```python
from build123d import *

# Parameters (mm, degrees)
ESQUISSE1_W                = 45
ESQUISSE1_H                = 13
BOSS_EXTRU_1_DEPTH         = 3
ESQUISSE2_R                = 1.5
ENL_V_MAT_EXTRU_1_DEPTH    = 4
BOSS_EXTRU_3_DEPTH         = 100
CONG_1_R                   = 1
ESQUISSE12_R               = 2.25
ENL_V_MAT_EXTRU_3_DEPTH    = 11.149508308
R_P_TITION_LIN_AIRE1_COUNT = 2
R_P_TITION_LIN_AIRE1_PITCH = 16


with BuildPart() as part:
    # Esquisse1 → Boss.-Extru.1 (new body)
    with BuildSketch(Plane.XY):
        with Locations((22.5, 6.5)):
            Rectangle(ESQUISSE1_W, ESQUISSE1_H)
    extrude(amount=BOSS_EXTRU_1_DEPTH)

    # Esquisse2 → Enl_v. mat.-Extru.1 (cut, through all)
    with BuildSketch(Plane.XY.offset(3)):
        with Locations((41, 6.5)):
            Circle(ESQUISSE2_R)
    enl_v_mat_extru_1 = extrude(amount=-ENL_V_MAT_EXTRU_1_DEPTH, mode=Mode.SUBTRACT)

    # Sym_trie1: Enl_v. mat.-Extru.1 across plane
    add(enl_v_mat_extru_1.mirror(Plane.ZY.offset(-22.5)), mode=Mode.SUBTRACT)

    # Esquisse8 → Boss.-Extru.3 (add)
    with BuildSketch(Plane.ZY):
        Polygon((0, 13), (-3.069268098, 21.432744793), (-0.420201433, 22.396926208), (3, 13), align=None)
    extrude(amount=-BOSS_EXTRU_3_DEPTH)

    # Cong_1
    cong_1_edges = [part.edges().sort_by_distance(p)[0] for p in [
        (45, 0, 1.5),
        (0, 0, 1.5),
        (45, 13, 1.5),
        (100, 13, 1.5),
        (100, 21.914835501, -1.744734766),
        (0, 21.914835501, -1.744734766),
    ]]
    fillet(cong_1_edges, radius=CONG_1_R)

    # Esquisse12 → Enl_v. mat.-Extru.3 (cut, through all)
    with BuildSketch(Plane(origin=(0, 2.484892534, 6.827186128), x_dir=(1, 0, 0), z_dir=(0, 0.342020143, 0.939692621))):
        with Locations((95, 15.68994364)):
            Circle(ESQUISSE12_R)
    enl_v_mat_extru_3 = extrude(amount=-ENL_V_MAT_EXTRU_3_DEPTH, mode=Mode.SUBTRACT)

    # R_p_tition lin_aire1: Enl_v. mat.-Extru.3 ×2
    with Locations(*[(-i * R_P_TITION_LIN_AIRE1_PITCH, 0, 0) for i in range(1, R_P_TITION_LIN_AIRE1_COUNT)]):
        add(enl_v_mat_extru_3, mode=Mode.SUBTRACT)


solid = part.part
```
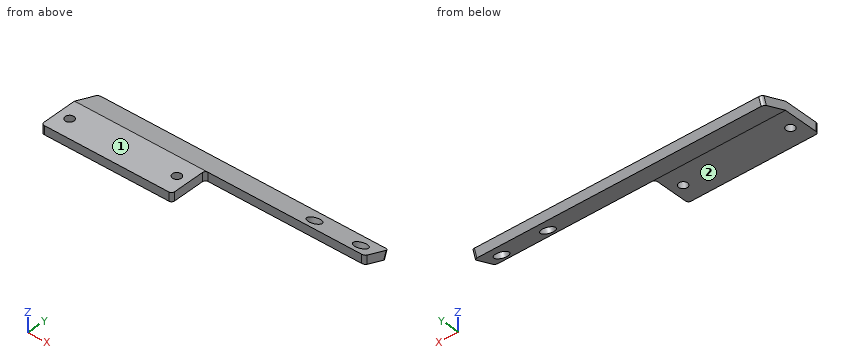
Part model, mm, in its own coordinate system. Face numbers are marked on the shaded views. A direction names the side the tool comes from. Coordinates: 2 decimals unless noted, no trailing zeros. Order: outer loops, then holes, each group sorted by start corner. A loop starts at its lowest first (then second) coordinate and runs counter-clockwise, first axis right, second up. Notation, with made-up numbers: (-20, 38.5) -> (7, 38.5) arc R38 cw to (7, 77.5) -> close; hole circle Ø5 at (-39, 30). An arc over 180 degrees is marked (long way). Put each result on its own line as item: value. Start each with the question number.
(1) Probe line 1 along X through (y, z) = (16.5, 1.25); line 2 along X through (y, z) = (11, 1.75); line 3 along Z through (x, y) = (9, 3). List the from-to ranges inside material, lowest first. Write a range as [from, to].
(2) Pin check, flat tips, straight feed: pin 1 Ø3.5 at (y, z) = (6.5, 1) entering from +X; pin 2 Ø1.5 at (x, y) = (26.5, 8) entering from -Z; pin 3 Ø2.5 at (x, z) = (69, 1.5) entering from -Y; pin 4 Ø1.8 at (x, y) = (41, 6.5) entering from +Z. Stop position of each tip, or through.
(3) Band-saw the part on B-B (y = 6.5). Give the cut face in (x, z), then the cut area to 3 significant figures.
(4) Band-saw the part on C-C (x = 86). Give the cut face in (y, z).
(5) Band-saw the part on A-A (x = 4). Give the cut face in (y, z).
(6) Which spindle directions (+Z, -Z, +X, -X, +Y, -Y) get a long thin tool onto all of the face, cutting with end or side? Do the marked faces 1 and 2. Say none if no direction does.
Determined:
1. line 1: x = [0, 76.83], [81.17, 92.83], [97.17, 100]
1. line 2: x = [0, 45]
1. line 3: z = [0, 3]
2. pin 1: stops at x = 45
2. pin 2: stops at z = 0
2. pin 3: stops at y = 13
2. pin 4: passes through
3. outline: (0, 0) -> (2.5, 0) -> (2.5, 3) -> (0, 3) -> close; (5.5, 0) -> (39.5, 0) -> (39.5, 3) -> (5.5, 3) -> close; (42.5, 0) -> (45, 0) -> (45, 3) -> (42.5, 3) -> close
3. area: 117 mm²
4. outline: (13, 0) -> (21.43, -3.07) -> (22.4, -0.42) -> (13, 3) -> close
5. outline: (0, 0) -> (5, 0) -> (5, 3) -> (0, 3) -> close; (8, 0) -> (13, 0) -> (21.43, -3.07) -> (22.4, -0.42) -> (13, 3) -> (8, 3) -> close
6. face 1: +Z, +X, -X, +Y, -Y
6. face 2: -Z, +X, -X, -Y
